The model under review builds one solid part; all positions refer to its coordinate system, in mm. Face numbers are marked on the shaded views. A direction names the side the tool comes from. Coordinates: 2 decimals unless noted, no trailing zeros. Write each loop counter-clockwise with the first axis right and the second up, starting at its lowest first coordinate (ties: lowest second). Pieces come first, ordered by that corner, then holes. Notation, with made-up numbers: (-11.75, 77.5) - (0.25, 77.5) arc R25 cw to (0.25, 112.5) - close; hole circle Ø11 at (50.25, 59.5). An arc over 180 degrees is marked (long way). Return JSON: item names as keys, results as strings. Group by question number.
(1) Draft analysis for pull direction X (two halves, no side actions). For the marked faces 1, 2, 3 and 4, state which applies: released by +X, released by -X, zero draft, split by the parting line, or undercut.
(2) We need section A-A on x = 0. State the section outline as (y, z) points.
(3) We need section D-D on y = -6.5. State the section outline as (x, z) points.
(4) For pin 1 Ø15 at (x, y) = (-2, 4.5) entering from +Z; pin 2 Ø4 at (x, z) = (-15, 4.5) entering from -Y; pin 3 Ø1.5 at (x, z) = (3, 1.5) entering from -Y; pin 4 Ø3.5 at (x, y) = (19.57, 0) entering from -Z, all flat-tipped, find the tip position at first contact; note any pin that passes through.
(5) To check wall thickness, follow L1, parallel to Y at x = 0, z = 9.3; L2, parallel to Z at x = 12, y = -17; L3, parallel to X at y = -9.5, z = 6.5. State the ranges of each line that lie inside material, in increasing order. Write a range as from..to.
(6) We need section B-B on y = 0. State the section outline as (x, z) points.
(7) We need section C-C on z = 4.25. State the section outline as (x, y) points, then the cut area to 3 significant figures.
(8) Tool access review of the marked faces 5 and 6: name each direction out of +Z, -Z, +X, -X, +Y, -Y from which nothing blocks a thin tool from reaching the whole face with its end or side.
```python
from build123d import *

# Parameters (mm, degrees)
SKIZZE1_R                       = 25
AUFSATZ_LINEAR_AUSTRAGEN1_DEPTH = 9
SKIZZE3_R                       = 25
SKIZZE3_R_2                     = 24
AUFSATZ_LINEAR_AUSTRAGEN2_DEPTH = 1
SCHNITT_LINEAR_AUSTRAGEN1_REACH = 38.483
SKIZZE4_W                       = 15.2
SKIZZE4_H                       = 20.2
SKIZZE6_R                       = 25
SKIZZE6_R_2                     = 23
SCHNITT_LINEAR_AUSTRAGEN2_DEPTH = 6
SKIZZE7_R                       = 1.5
SCHNITT_LINEAR_AUSTRAGEN3_DEPTH = 37.742346142
SKIZZE8_R                       = 1.5
SCHNITT_LINEAR_AUSTRAGEN4_DEPTH = 37.742346142


with BuildPart() as part:
    # Skizze1 → Aufsatz-Linear austragen1 (new body)
    with BuildSketch(Plane.XY):
        Circle(SKIZZE1_R)
    extrude(amount=AUFSATZ_LINEAR_AUSTRAGEN1_DEPTH)

    # Skizze3 → Aufsatz-Linear austragen2 (add)
    with BuildSketch(Plane.XY.offset(9)):
        Circle(SKIZZE3_R)
        Circle(SKIZZE3_R_2, mode=Mode.SUBTRACT)
    extrude(amount=AUFSATZ_LINEAR_AUSTRAGEN2_DEPTH)

    # Skizze4 → Schnitt-Linear austragen1 (cut, up to next)
    with BuildSketch(Plane.XY.offset(9), mode=Mode.PRIVATE) as schnitt_linear_austragen1_sk1:
        with Locations((0.09, 0)):
            Rectangle(SKIZZE4_W, SKIZZE4_H)
    schnitt_linear_austragen1_tool1 = extrude(schnitt_linear_austragen1_sk1.sketch, amount=-SCHNITT_LINEAR_AUSTRAGEN1_REACH, mode=Mode.PRIVATE) & part.part
    add(schnitt_linear_austragen1_tool1.solids().sort_by_distance((0.09, 0, 9))[0], mode=Mode.SUBTRACT)

    # Skizze6 → Schnitt-Linear austragen2 (cut)
    with BuildSketch(Plane(origin=(0, 0, 2), x_dir=(-1, 0, 0), z_dir=(0, 0, -1))):
        Circle(SKIZZE6_R)
        Circle(SKIZZE6_R_2, mode=Mode.SUBTRACT)
    extrude(amount=-SCHNITT_LINEAR_AUSTRAGEN2_DEPTH, mode=Mode.SUBTRACT)

    # Skizze7 → Schnitt-Linear austragen3 (cut, through all)
    with BuildSketch(Plane(origin=(0, 0, 0), x_dir=(-1, 0, 0), z_dir=(0, 0, -1))):
        with Locations((-19.569472829, 0)):
            Circle(SKIZZE7_R)
    extrude(amount=-SCHNITT_LINEAR_AUSTRAGEN3_DEPTH, mode=Mode.SUBTRACT)

    # Skizze8 → Schnitt-Linear austragen4 (cut, through all)
    with BuildSketch(Plane(origin=(0, 0, 0), x_dir=(-1, 0, 0), z_dir=(0, 0, -1))):
        with Locations((-25, 0)):
            Circle(SKIZZE8_R)
    extrude(amount=-SCHNITT_LINEAR_AUSTRAGEN4_DEPTH, mode=Mode.SUBTRACT)


solid = part.part
```
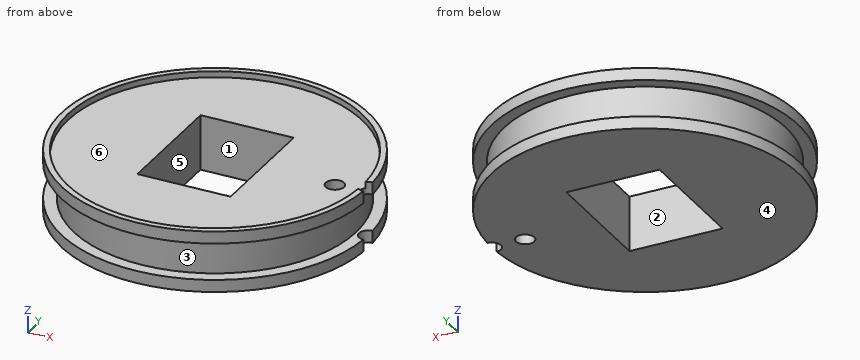
Ans:
{
 "1": {"face 1": "undercut", "face 2": "undercut", "face 3": "split by the parting line", "face 4": "zero draft"},
 "2": {"outline": "(-25, 0) - (-10.1, 0) - (-10.1, 9) - (-24, 9) - (-24, 10) - (-25, 10) - (-25, 8) - (-23, 8) - (-23, 2) - (-25, 2) - close; (10.1, 0) - (25, 0) - (25, 2) - (23, 2) - (23, 8) - (25, 8) - (25, 10) - (24, 10) - (24, 9) - (10.1, 9) - close"},
 "3": {"outline": "(-24.14, 0) - (-7.51, 0) - (-7.51, 9) - (-23.1, 9) - (-23.1, 10) - (-24.14, 10) - (-24.14, 8) - (-22.06, 8) - (-22.06, 2) - (-24.14, 2) - close; (7.69, 0) - (24.14, 0) - (24.14, 2) - (22.06, 2) - (22.06, 8) - (24.14, 8) - (24.14, 10) - (23.1, 10) - (23.1, 9) - (7.69, 9) - close"},
 "4": {"pin 1": "z = 9", "pin 2": "y = -18.97", "pin 3": "y = -24.9", "pin 4": "z = 0"},
 "5": {"L1": "-25..-24, 24..25", "L2": "0..9", "L3": "-20.95..-7.51, 7.69..20.95"},
 "6": {"outline": "(-25, 0) - (-7.51, 0) - (-7.51, 9) - (-24, 9) - (-24, 10) - (-25, 10) - (-25, 8) - (-23, 8) - (-23, 2) - (-25, 2) - close; (7.69, 0) - (18.07, 0) - (18.07, 9) - (7.69, 9) - close; (21.07, 0) - (23.5, 0) - (23.5, 2) - (23, 2) - (23, 8) - (23.5, 8) - (23.5, 9) - (21.07, 9) - close"},
 "7": {"outline": "circle Ø46 at (0, 0); hole (-7.51, -10.1) - (7.69, -10.1) - (7.69, 10.1) - (-7.51, 10.1) - close; hole circle Ø3 at (19.57, 0)", "area": "1,350 mm²"},
 "8": {"face 5": "+Z, -Z", "face 6": "+Z"}
}
